Design review of the part built by this model. Coordinates are the model's own, in mm. Round coordinates to 2 decimals unless told otherwise and drop trailing zeros. Loops run counter-clockwise (first coordinate to the right, second up) from the corner with the lowest first, then second, coordinate; pieces in that order, holes last. Notation, with made-up numbers: M 62,4.25 L 101,4.25 A30 cw 101,42.25 Z; hole C 2.5,-35.75 d4. An arc over 180 degrees is marked long. Use a Markdown table: item, result.
from build123d import *

# Parameters (mm, degrees)
SKETCH1_W           = 90
SKETCH1_H           = 140
SKETCH1_R           = 5
SKETCH1_R_2         = 2.1
BOSS_EXTRUDE1_DEPTH = 3


with BuildPart() as part:
    # Sketch1 → Boss-Extrude1 (new body)
    with BuildSketch(Plane(origin=(0, 0, 0), x_dir=(0, 0, -1), z_dir=(1, 0, 0))):
        with Locations((45, -70)):
            Rectangle(SKETCH1_W, SKETCH1_H)
        with Locations((34, -70)):
            Circle(SKETCH1_R, mode=Mode.SUBTRACT)
        with Locations((34, -45)):
            Circle(SKETCH1_R_2, mode=Mode.SUBTRACT)
        with Locations((55.650635095, -82.5)):
            Circle(SKETCH1_R_2, mode=Mode.SUBTRACT)
        with Locations((12.349364905, -82.5)):
            Circle(SKETCH1_R_2, mode=Mode.SUBTRACT)
        with Locations((9, -6)):
            Circle(SKETCH1_R_2, mode=Mode.SUBTRACT)
        with Locations(Location((81, -6, 0), (0, 0, 180))):
            Circle(SKETCH1_R_2, mode=Mode.SUBTRACT)
        with Locations((81, -134)):
            Circle(SKETCH1_R_2, mode=Mode.SUBTRACT)
        with Locations(Location((9, -134, 0), (0, 0, 180))):
            Circle(SKETCH1_R_2, mode=Mode.SUBTRACT)
        with BuildLine():
            Line((34, -90.5), (28.5, -90.5))
            ThreePointArc((28.5, -90.5), (27.085786438, -91.085786438), (26.5, -92.5))
            Line((26.5, -92.5), (26.5, -96.5))
            ThreePointArc((26.5, -96.5), (27.085786438, -97.914213562), (28.5, -98.5))
            Line((28.5, -98.5), (39.5, -98.5))
            ThreePointArc((39.5, -98.5), (40.914213562, -97.914213562), (41.5, -96.5))
            Line((41.5, -96.5), (41.5, -92.5))
            ThreePointArc((41.5, -92.5), (40.914213562, -91.085786438), (39.5, -90.5))
            Line((39.5, -90.5), (34, -90.5))
        make_face(mode=Mode.SUBTRACT)
    extrude(amount=BOSS_EXTRUDE1_DEPTH)


solid = part.part
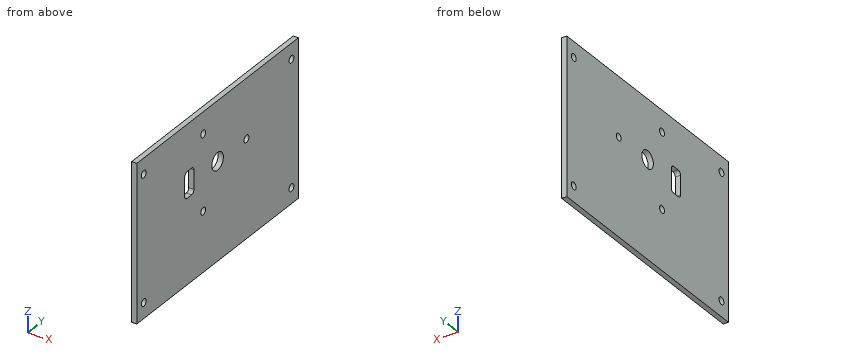
1. Take a section at A-A on y = -82.5. Give the boundary of the cut face in (x, z), and give its area (3 significant figures).
Check values:
| item | result |
|---|---|
| outline | M 0,-90 L 3,-90 L 3,-57.75 L 0,-57.75 Z; M 0,-53.55 L 3,-53.55 L 3,-14.45 L 0,-14.45 Z; M 0,-10.25 L 3,-10.25 L 3,0 L 0,0 Z |
| area | 245 mm² |
2. Take a section at C-C on z = -81. Give the boundary of the cut face in (x, y).
Check values:
| item | result |
|---|---|
| outline | M 0,-140 L 3,-140 L 3,-136.1 L 0,-136.1 Z; M 0,-131.9 L 3,-131.9 L 3,-8.1 L 0,-8.1 Z; M 0,-3.9 L 3,-3.9 L 3,0 L 0,0 Z |
3. Take a section at D-D on z = -34. Give the boundary of the cut face in (x, y).
Check values:
| item | result |
|---|---|
| outline | M 0,-140 L 3,-140 L 3,-98.5 L 0,-98.5 Z; M 0,-90.5 L 3,-90.5 L 3,-75 L 0,-75 Z; M 0,-65 L 3,-65 L 3,-47.1 L 0,-47.1 Z; M 0,-42.9 L 3,-42.9 L 3,0 L 0,0 Z |
4. Wall thickness on line 1 along Y through (x, z) = (1.9, -34); line 2 along Y through (x, z) = (1.3, -9); line 3 along Z through (x, y) = (1.6, -134): over which ranges is each line inside the solid? List them lowest first. Write a range as from..to.
Check values:
| item | result |
|---|---|
| line 1 | y = -140..-98.5, -90.5..-75, -65..-47.1, -42.9..0 |
| line 2 | y = -140..-136.1, -131.9..-8.1, -3.9..0 |
| line 3 | z = -90..-83.1, -78.9..-11.1, -6.9..0 |
5. Insertion check: pin 1 (2.5 mm diameter, centred on y = -6, z = -9, fed in from -X). The pin has a flat end and moves straight along its axis. Give the tip position at first contact, or say it passes through.
Check values:
| item | result |
|---|---|
| pin 1 | passes through |
6. Take a section at B-B on y = -45. Give the boundary of the cut face in (x, z), and give its area (3 significant figures).
Check values:
| item | result |
|---|---|
| outline | M 0,-90 L 3,-90 L 3,-36.1 L 0,-36.1 Z; M 0,-31.9 L 3,-31.9 L 3,0 L 0,0 Z |
| area | 257 mm² |
